Work out the finished part from the listing and answer in its coordinate system (mm). Face numbers are marked on the shaded views. A direction names the side the tool comes from. Coordinates: 2 decimals unless noted, no trailing zeros. Order: outer loops, then holes, each group sorted by start corner. A loop starts at its lowest first (then second) coordinate and runs counter-clockwise, first axis right, second up.
Autodesk Inventor part; units mm, degrees
ref_plane "YZ Plane" through (0, 0, 0) normal (1, 0, 0) x (0, 1, 0)
ref_plane "XZ Plane" through (0, 0, 0) normal (0, 1, 0) x (-1, 0, 0)
ref_plane "XY Plane" through (0, 0, 0) normal (0, 0, 1) x (1, 0, 0)
sketch "Sketch1" plane through (0, 0, 0) normal (0, 0, 1) x (1, 0, 0)
  circle A0 centre (0, 0) radius 8 construction
  circle A1 centre (0, 0) radius 16 construction
  line L0 (20, -8.2843) -> (8.2843, -20)
  line L1 (8.2843, -20) -> (-8.2843, -20)
  line L2 (-8.2843, -20) -> (-20, -8.2843)
  line L3 (-20, 8.2843) -> (-8.2843, 20)
  line L4 (-8.2843, 20) -> (8.2843, 20)
  line L5 (8.2843, 20) -> (20, 8.2843)
  line L6 (20, 8.2843) -> (20, -8.2843)
  line L7 (-7.7279, 5) -> (-20, 5)
  line L8 (-7.7279, -5) -> (-20, -5)
  circle A2 centre (0, 0) radius 4.2
  line L9 (-20, -8.2843) -> (-20, -5)
  line L10 (-20, 5) -> (-20, 8.2843)
  line L11 (28, -11.598) -> (11.598, -28)
  line L12 (11.598, -28) -> (-11.598, -28)
  line L13 (-11.598, -28) -> (-28, -11.598)
  line L14 (-28, -11.598) -> (-28, 11.598)
  line L15 (-28, 11.598) -> (-11.598, 28)
  line L16 (-11.598, 28) -> (11.598, 28)
  line L17 (11.598, 28) -> (28, 11.598)
  line L18 (28, 11.598) -> (28, -11.598)
  line L19 (9, -3.7279) -> (3.7279, -9)
  line L20 (3.7279, -9) -> (-3.7279, -9)
  line L21 (-3.7279, 9) -> (3.7279, 9)
  line L22 (3.7279, 9) -> (9, 3.7279)
  line L23 (9, 3.7279) -> (9, -3.7279)
  line L24 (-20, 5) -> (-20, -5) construction
  line L25 (-3.7279, 9) -> (-7.7279, 5)
  line L26 (-3.7279, -9) -> (-7.7279, -5)
  point P0 (-20, 0)
  dimension "d1" = 16
  dimension "d2" = 32
  dimension "d5" = 8.4
  dimension "d6" = 40
  dimension "d7" = 8
  dimension "d8" = 10
  dimension "d10" = 18
extrude "Extrusion1" add sketch "Sketch1" along normal blind 6
sketch "Sketch2" plane through (0, 0, 6) normal (0, 0, 1) x (1, 0, 0)
  circle A0 centre (0, 0) radius 4.2
  line L0 (11.598, 28) -> (-11.598, 28)
  line L1 (-11.598, 28) -> (-28, 11.598)
  line L2 (-28, 11.598) -> (-28, -11.598)
  line L3 (-28, -11.598) -> (-11.598, -28)
  line L4 (-11.598, -28) -> (11.598, -28)
  line L5 (-24.7487, 14.8492) -> (-28, 18.1005)
  line L6 (-28, 18.1005) -> (-28, 23.8995)
  line L7 (-28, 23.8995) -> (-23.8995, 28)
  line L8 (-23.8995, 28) -> (-18.1005, 28)
  line L9 (-18.1005, 28) -> (-14.8492, 24.7487)
  line L10 (-28, 21) -> (-21, 21) construction
  line L11 (-21, 28) -> (-21, 21) construction
  circle A1 centre (-21, 21) radius 3.2
  line L12 (-24.7487, 14.8492) -> (-14.8492, 24.7487)
  line L13 (-14.8492, -24.7487) -> (-18.1005, -28)
  line L14 (-18.1005, -28) -> (-23.8995, -28)
  line L15 (-23.8995, -28) -> (-28, -23.8995)
  line L16 (-28, -23.8995) -> (-28, -18.1005)
  line L17 (-28, -18.1005) -> (-24.7487, -14.8492)
  circle A2 centre (-21, -21) radius 3.2
  line L18 (-14.8492, -24.7487) -> (-24.7487, -14.8492)
  line L19 (24.7487, -14.8492) -> (28, -18.1005)
  line L20 (28, -18.1005) -> (28, -23.8995)
  line L21 (28, -23.8995) -> (23.8995, -28)
  line L22 (23.8995, -28) -> (18.1005, -28)
  line L23 (18.1005, -28) -> (14.8492, -24.7487)
  circle A3 centre (21, -21) radius 3.2
  line L24 (24.7487, -14.8492) -> (14.8492, -24.7487)
  line L25 (14.8492, 24.7487) -> (18.1005, 28)
  line L26 (18.1005, 28) -> (23.8995, 28)
  line L27 (23.8995, 28) -> (28, 23.8995)
  line L28 (28, 23.8995) -> (28, 18.1005)
  line L29 (28, 18.1005) -> (24.7487, 14.8492)
  circle A4 centre (21, 21) radius 3.2
  line L30 (14.8492, 24.7487) -> (24.7487, 14.8492)
  circle A5 centre (-21, 21) radius 6 construction
  point P0 (-19.799, 19.799)
  point P1 (-21, -28)
  point P2 (-28, -21)
  point P3 (28, -21)
  point P4 (21, -28)
  point P5 (21, 28)
  point P6 (28, 21)
  dimension "d13" = 14
  dimension "d14" = 7
  dimension "d15" = 6.4
  dimension "d18" = 360
  dimension "d22" = 12
extrude "Extrusion2" add sketch "Sketch2" against normal blind 6 contours L3 A2 L13 L14 L15 L16 L17 | L5 L6 L7 L8 L9 L1 A1 | L19 L20 L21 L22 L23 L24 A3 | L25 L26 L27 L28 L29 L30 A4
sketch "Sketch3" plane through (0, 0, 6) normal (0, 0, 1) x (1, 0, 0)
  line L0 (-17.8813, 21.7167) -> (-21.7167, 17.8813)
  arc A0 (-17.8813, 21.7167) -> (-21.7167, 17.8813) centre (-21, 21) ccw
  line L1 (-21.7167, -17.8813) -> (-17.8813, -21.7167)
  arc A1 (-21.7167, -17.8813) -> (-17.8813, -21.7167) centre (-21, -21) ccw
  arc A2 (17.8813, -21.7167) -> (21.7167, -17.8813) centre (21, -21) ccw
  line L2 (17.8813, -21.7167) -> (21.7167, -17.8813)
  arc A3 (21.7167, 17.8813) -> (17.8813, 21.7167) centre (21, 21) ccw
  line L3 (21.7167, 17.8813) -> (17.8813, 21.7167)
  circle A4 centre (-21, -21) radius 3.2
  circle A5 centre (-21, 21) radius 3.2
  circle A6 centre (21, 21) radius 3.2
  circle A7 centre (21, -21) radius 3.2
extrude "Extrusion3" cut sketch "Sketch3" against normal through all contours A5 L0 | A4 L1 | A7 L2 | A6 L3
sketch "Sketch4" plane through (0, 0, 0) normal (0, 0, -1) x (-1, 0, 0)
  circle A0 centre (21, -21) radius 3.2
  circle A1 centre (21, 21) radius 3.2
  circle A2 centre (-21, -21) radius 3.2
  line L0 (-24.7487, -14.8492) -> (-28, -18.1005)
  line L1 (-28, -18.1005) -> (-28, -23.8995)
  line L2 (-28, -23.8995) -> (-23.8995, -28)
  line L3 (-23.8995, -28) -> (-18.1005, -28)
  line L4 (-18.1005, -28) -> (-14.8492, -24.7487)
  line L5 (-14.8492, -24.7487) -> (-11.598, -28)
  line L6 (-11.598, -28) -> (11.598, -28)
  line L7 (11.598, -28) -> (14.8492, -24.7487)
  line L8 (14.8492, -24.7487) -> (18.1005, -28)
  line L9 (18.1005, -28) -> (23.8995, -28)
  line L10 (23.8995, -28) -> (28, -23.8995)
  line L11 (28, -23.8995) -> (28, -18.1005)
  line L12 (28, -18.1005) -> (24.7487, -14.8492)
  line L13 (24.7487, -14.8492) -> (28, -11.598)
  line L14 (28, -11.598) -> (28, 11.598)
  line L15 (28, 11.598) -> (24.7487, 14.8492)
  line L16 (24.7487, 14.8492) -> (28, 18.1005)
  line L17 (28, 18.1005) -> (28, 23.8995)
  line L18 (28, 23.8995) -> (23.8995, 28)
  line L19 (23.8995, 28) -> (18.1005, 28)
  line L20 (18.1005, 28) -> (14.8492, 24.7487)
  line L21 (14.8492, 24.7487) -> (11.598, 28)
  line L22 (11.598, 28) -> (-11.598, 28)
  line L23 (-11.598, 28) -> (-14.8492, 24.7487)
  line L24 (-14.8492, 24.7487) -> (-18.1005, 28)
  line L25 (-18.1005, 28) -> (-23.8995, 28)
  line L26 (-23.8995, 28) -> (-28, 23.8995)
  line L27 (-28, 23.8995) -> (-28, 18.1005)
  line L28 (-28, 18.1005) -> (-24.7487, 14.8492)
  line L29 (-24.7487, 14.8492) -> (-28, 11.598)
  line L30 (-28, 11.598) -> (-28, -11.598)
  line L31 (-28, -11.598) -> (-24.7487, -14.8492)
  circle A3 centre (-21, 21) radius 3.2
  line L32 (8.2843, -20) -> (-8.2843, -20)
  line L33 (-8.2843, -20) -> (-20, -8.2843)
  line L34 (-20, -8.2843) -> (-20, 8.2843)
  line L35 (-20, 8.2843) -> (-8.2843, 20)
  line L36 (-8.2843, 20) -> (8.2843, 20)
  line L37 (8.2843, 20) -> (20, 8.2843)
  line L38 (20, 8.2843) -> (20, 5)
  line L39 (20, 5) -> (7.7279, 5)
  line L40 (7.7279, 5) -> (3.7279, 9)
  line L41 (3.7279, 9) -> (-3.7279, 9)
  line L42 (-3.7279, 9) -> (-9, 3.7279)
  line L43 (-9, 3.7279) -> (-9, -3.7279)
  line L44 (-9, -3.7279) -> (-3.7279, -9)
  line L45 (-3.7279, -9) -> (3.7279, -9)
  line L46 (3.7279, -9) -> (7.7279, -5)
  line L47 (7.7279, -5) -> (20, -5)
  line L48 (20, -5) -> (20, -8.2843)
  line L49 (20, -8.2843) -> (8.2843, -20)
  circle A4 centre (0, 0) radius 4.2
extrude "Extrusion4" add sketch "Sketch4" along normal blind 0.5
properties part number "x_iddler_belt_bearing_mount"
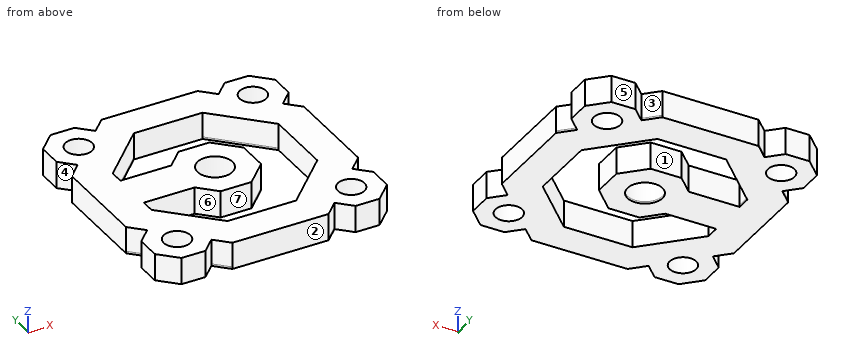
1. The part is cut by section C-C (x = 0). Determine the outline of the cut face in (y, z).
2. The mould has two halves that part along X. Classify the marked faces 4, 5, 6 and 7: released by +X, released by -X, zero draft, split by the parting line, or undercut.
3. Consider probe 1 along Y at (x, z) = (21, 3); probe 2 along X at (y, z) = (0, 3.05). Determine where each line is inside the solid, lowest interval first.
4. The part is cut by section B-B (y = 0). Determine the outline of the cut face in (x, z), plus the area to 3 significant figures.
5. The part is cut by section A-A (x = -21). Determine the outline of the cut face in (y, z).
6. A flat-ended cylindrical pin translates along its axis: pin 1 (1 mm diameter, centred on x = 27, y = 13.5, fed in from -Z). Find the tip coordinate at first contact, or state that the pin passes through.
7. For the marked faces 1, 2 and 3, determine the directions among +Z, -Z, +X, -X, +Y, -Y from which every point of the face is accessible in a straight line to the end or side of a thin tool.
Worked out:
1. outline: (-28, -0.5) - (-20, -0.5) - (-20, 6) - (-28, 6) - close; (-9, -0.5) - (-4.2, -0.5) - (-4.2, 6) - (-9, 6) - close; (4.2, -0.5) - (9, -0.5) - (9, 6) - (4.2, 6) - close; (20, -0.5) - (28, -0.5) - (28, 6) - (20, 6) - close
2. face 4: released by -X
2. face 5: zero draft
2. face 6: undercut
2. face 7: undercut
3. probe 1: y = -28 to -24.2, -17.8 to 17.8, 24.2 to 28
3. probe 2: x = -28 to -4.2, 4.2 to 9, 20 to 28
4. outline: (-28, -0.5) - (-4.2, -0.5) - (-4.2, 6) - (-28, 6) - close; (4.2, -0.5) - (9, -0.5) - (9, 6) - (4.2, 6) - close; (20, -0.5) - (28, -0.5) - (28, 6) - (20, 6) - close
4. area: 238 mm2
5. outline: (-28, -0.5) - (-24.2, -0.5) - (-24.2, 6) - (-28, 6) - close; (-17.8, -0.5) - (17.8, -0.5) - (17.8, 6) - (-17.8, 6) - close; (24.2, -0.5) - (28, -0.5) - (28, 6) - (24.2, 6) - close
6. pin 1: passes through
7. face 1: +Z, -Z
7. face 2: +Z, -Z, +X, -X, -Y
7. face 3: +Z, -Z, +Y
